Study the drawing (mm; zero at the part's minimum x, y, z) and answer. A direction names the side the tool comes from. Round coordinates to 2 decimals unless told otherwise and drop trailing zeros. Order: outer loops, then holes, each group sorted by start corner. A loop starts at its lowest first (then second) coordinate and runs counter-clockwise, first axis right, second up. Notation, with made-up numbers: (77, 45) -> (97, 45) arc R15 cw to (97, 54) -> close; hole circle Ø8 at (-31.5, 58.25). An arc over 180 degrees is marked (long way). Use one line per item in the form item = value.
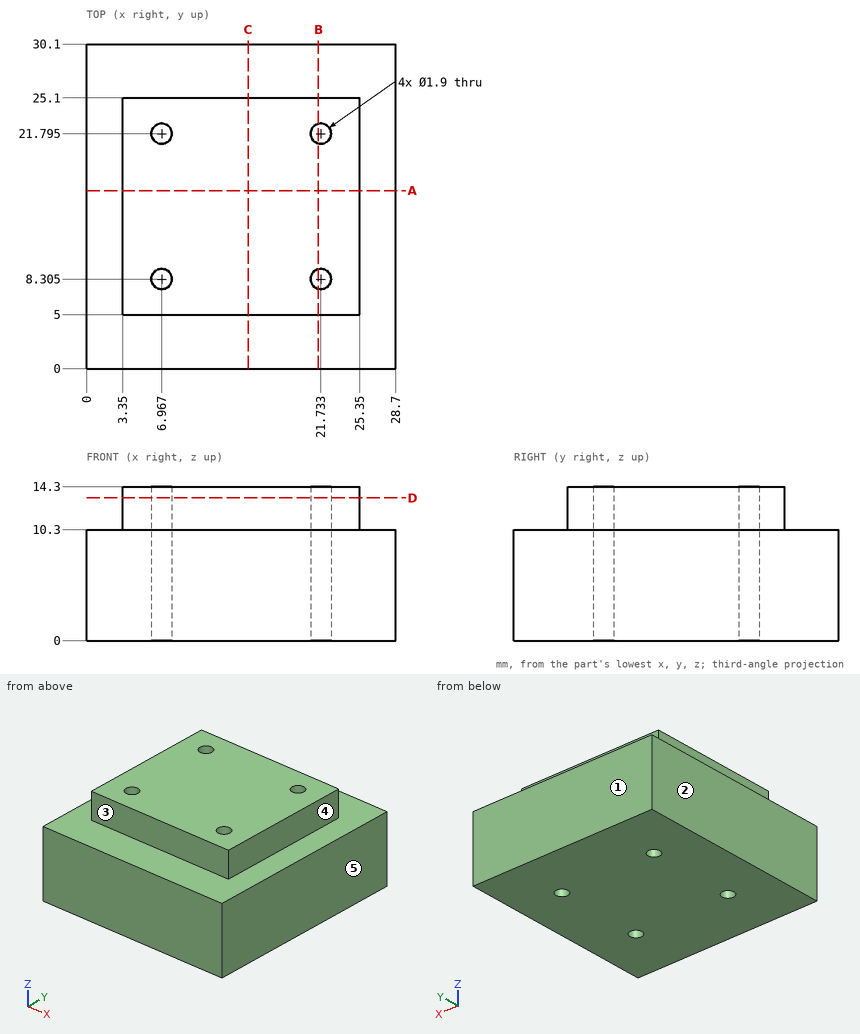
Item 1: Determine the mould class of the marked faces 1, 2 and 3 for opening direction Y: released by +Y, released by -Y, zero draft, split by the parting line, or undercut.
Findings:
face_1 = released by +Y
face_2 = zero draft
face_3 = released by -Y
Item 2: The part is cut by section C-C, the plane x = 15. Give the vertices of the cut face in (y, z).
Findings:
outline = (0, 0) -> (30.1, 0) -> (30.1, 10.3) -> (25.1, 10.3) -> (25.1, 14.3) -> (5, 14.3) -> (5, 10.3) -> (0, 10.3) -> close
Item 3: The part is cut by section A-A, the plane y = 16.5. Give the vertices of the cut face in (x, z), and give its area (3 significant figures).
Findings:
outline = (0, 0) -> (28.7, 0) -> (28.7, 10.3) -> (25.35, 10.3) -> (25.35, 14.3) -> (3.35, 14.3) -> (3.35, 10.3) -> (0, 10.3) -> close
area = 384 mm^2
Item 4: The part is cut by section D-D, the plane z = 13.25. Give the number of separate pieces and of enclosed holes in the cut face, and give its area (3 significant figures).
Findings:
separate_pieces = 1
enclosed_holes = 4
area = 431 mm^2
Item 5: Consider line 1 along X through (y, z) = (22.5, 9) (1 decimal); line 2 along Y through (x, z) = (21.5, 2) (1 decimal); line 3 along Z through (x, y) = (7.5, 26). Determine where each line is inside the solid, lowest interval first.
Findings:
line_1 = 0 to 6.3, 7.6 to 21.1, 22.4 to 28.7
line_2 = 0 to 7.4, 9.2 to 20.9, 22.7 to 30.1
line_3 = 0 to 10.3
Item 6: The part is cut by section B-B, the plane x = 21.5. Give the vertices of the cut face in (y, z), and give its area (3 significant figures).
Findings:
outline = (0, 0) -> (7.38, 0) -> (7.38, 14.3) -> (5, 14.3) -> (5, 10.3) -> (0, 10.3) -> close; (9.23, 0) -> (20.87, 0) -> (20.87, 14.3) -> (9.23, 14.3) -> close; (22.72, 0) -> (30.1, 0) -> (30.1, 10.3) -> (25.1, 10.3) -> (25.1, 14.3) -> (22.72, 14.3) -> close
area = 338 mm^2
Item 7: Flat-ended cylindrical pins translate along their axes: P1, Ø1.2, axis at x = 11.5, z = 12.5, coming from the -Y side; P2, Ø2, axis at y = 19.5, z = 12.5, coming from the +X side. Find the tip coordinate at first contact, or state that the pin passes through.
Findings:
P1 = 5
P2 = 25.35
Item 8: For the marked faces 4 and 5, determine the directions among +Z, -Z, +X, -X, +Y, -Y from which every point of the face is accessible in a straight line to the end or side of a thin tool.
Findings:
face_4 = +Z, +X, +Y, -Y
face_5 = +Z, -Z, +X, +Y, -Y
